For this review, take the finished solid that the model builds, in its own axes (mm). A direction names the side the tool comes from. Coordinates: 2 decimals unless noted, no trailing zeros. Order: outer loops, then holes, each group sorted by start corner. A loop starts at its lowest first (then second) coordinate and runs counter-clockwise, first axis right, second up. Notation, with made-up numbers: (27.5, -35) -> (51.5, -35) arc R37 ccw to (51.5, 2) -> close; hole circle Ø11 at (-22, 71.5). An arc over 180 degrees is marked (long way). Answer as a JSON object with one key per item and string values. Group by question number.
1) Add section D-D, the plane z = 22. Write out the cut boundary in (x, y), then the cut area to 3 significant figures.
2) For pin 1 (3 mm diameter, centred on x = 1.5, y = -4, fed in from +Z); pin 2 (1.5 mm diameter, centred on x = -1, z = 17, fed in from +Y); pin 3 (2 mm diameter, centred on x = 0, z = 4, fed in from +Y), all flat-tipped, find the tip position at first contact; note any pin that passes through.
3) Machinability: for faces 1 (the flat face through (0, 11.006, 0)), 2 (the flat face through (2.5, -6.2, -6.2)), which of the approach directions +Z, -Z, +X, -X, +Y, -Y give a long, thin tool a straight path to every point of the face, cutting with its end or side? Answer none if there is none.
4) Draft analysis for pull direction Y (two halves, no side actions). For faces 3 (the cylindrical face through (0.04, 1.32, 29.97)), 4 (the flat face through (-2.5, -6.2, -6.2)), 5 (the flat face through (0, 10, 3)), state which applies: +Y half, -Y half, draft (parallel to the pull), parting line (faces both ways), or undercut.
5) Add section B-B, the plane z = 0. Write out the cut boundary in (x, y), then the cut area to 3 significant figures.
6) Add section C-C, the plane x = -0.95. Write out the cut boundary in (y, z), then the cut area to 3 significant figures.
7) Add section A-A, the plane y = 0. Write out the cut boundary in (x, z), then the cut area to 4 significant figures.
8) Wall thickness on L1, parallel to Y at x = 0, z = -7.5; L2, parallel to Y at x = 1.75, z = 2.5; L3, parallel to Z at x = -1.95, y = 8.5: over which ranges is each line inside the solid? List them lowest first.
from build123d import *

# Parameters (mm, degrees)
SKETCH1_R           = 30
BOSS_EXTRUDE1_DEPTH = 2.5
CUT_EXTRUDE4_DEPTH  = 43.720018727


with BuildPart() as part:
    # Sketch1 → Boss-Extrude1 (new, symmetric)
    with BuildSketch(Plane(origin=(0, 0, 0), x_dir=(0, 0, -1), z_dir=(1, 0, 0))):
        Circle(SKETCH1_R)
    extrude(amount=BOSS_EXTRUDE1_DEPTH, both=True)

    # Sketch8 → Cut-Extrude4 (cut, through all)
    with BuildSketch(Plane(origin=(2.5, 0, 0), x_dir=(0, 0, -1), z_dir=(1, 0, 0))):
        with BuildLine():
            Line((0, 11.006403687), (-3, 11.006403687))
            Line((-3, 11.006403687), (-3, 8.006403687))
            ThreePointArc((-3, 8.006403687), (0, -8.55), (3, 8.006403687))
            Line((3, 8.006403687), (3, 11.006403687))
            Line((3, 11.006403687), (0, 11.006403687))
        make_face()
    extrude(amount=-CUT_EXTRUDE4_DEPTH, mode=Mode.SUBTRACT)


solid = part.part
Output values:
{
 "1": {"outline": "(-2.5, -20.4) -> (2.5, -20.4) -> (2.5, 20.4) -> (-2.5, 20.4) -> close", "area": "204 mm²"},
 "2": {"pin 1": "stops at z = 29.9", "pin 2": "stops at y = 25.22", "pin 3": "stops at y = 29.85"},
 "3": {"face 1": "+X, -X", "face 2": "+Z, -Z, +X, +Y, -Y"},
 "4": {"face 3": "parting line", "face 4": "draft", "face 5": "undercut"},
 "5": {"outline": "(-2.5, -30) -> (2.5, -30) -> (2.5, -8.55) -> (-2.5, -8.55) -> close; (-2.5, 11.01) -> (2.5, 11.01) -> (2.5, 30) -> (-2.5, 30) -> close", "area": "202 mm²"},
 "6": {"outline": "circle Ø60 at (0, 0); hole (8.01, -3) -> (11.01, -3) -> (11.01, 3) -> (8.01, 3) arc R8.55 ccw (long way) to start", "area": "2,580 mm²"},
 "7": {"outline": "(-2.5, -30) -> (2.5, -30) -> (2.5, -8.55) -> (-2.5, -8.55) -> close; (-2.5, 8.55) -> (2.5, 8.55) -> (2.5, 30) -> (-2.5, 30) -> close", "area": "214.5 mm²"},
 "8": {"L1": "y = -29.05 to -4.11, 4.11 to 29.05", "L2": "y = -29.9 to -8.18, 11.01 to 29.9", "L3": "z = -28.77 to -3, 3 to 28.77"}
}
